from build123d import *

# Parameters (mm, degrees)
SKETCH_1_R          = 1.6
SKETCH_1_W          = 32
SKETCH_1_H          = 32
EXTRUDE_1_DEPTH     = 30
SKETCH_3_W          = 32
SKETCH_3_H          = 32
EXTRUDE_2_DEPTH     = 5
SKETCH_4_R          = 6.35
CUT_EXTRUDE_1_DEPTH = 53.250598083
SKETCH_5_R          = 10
CUT_EXTRUDE_2_DEPTH = 3
CUT_EXTRUDE_3_DEPTH = 3.5
EXTRUDE_3_DEPTH     = 60.5
SKETCH_14_W         = 12.25
SKETCH_14_H         = 14
SKETCH_14_R         = 1.6
EXTRUDE_4_DEPTH     = 4
EXTRUDE_5_DEPTH     = 3
FILLET_1_R          = 1


with BuildPart() as part:
    # ｽｹｯﾁ1 → ﾎﾞｽ - 押し出し1 (new body)
    with BuildSketch(Plane.XY):
        with BuildLine():
            Line((30.25, -30.25), (30.25, 27.25))
            ThreePointArc((30.25, 27.25), (29.371320344, 29.371320344), (27.25, 30.25))
            Line((27.25, 30.25), (-27.25, 30.25))
            ThreePointArc((-27.25, 30.25), (-29.371320344, 29.371320344), (-30.25, 27.25))
            Line((-30.25, 27.25), (-30.25, -30.25))
            Line((-30.25, -30.25), (30.25, -30.25))
        make_face()
        with Locations((-26.25, 26.25)):
            Circle(SKETCH_1_R, mode=Mode.SUBTRACT)
        with Locations((-26.25, -26.25)):
            Circle(SKETCH_1_R, mode=Mode.SUBTRACT)
        with Locations((26.25, -26.25)):
            Circle(SKETCH_1_R, mode=Mode.SUBTRACT)
        with Locations((26.25, 26.25)):
            Circle(SKETCH_1_R, mode=Mode.SUBTRACT)
        Rectangle(SKETCH_1_W, SKETCH_1_H, mode=Mode.SUBTRACT)
    extrude(amount=-EXTRUDE_1_DEPTH)

    # ｽｹｯﾁ3 → ﾎﾞｽ - 押し出し2 (add)
    with BuildSketch(Plane(origin=(0, 0, -30), x_dir=(-1, 0, 0), z_dir=(0, 0, -1))):
        Rectangle(SKETCH_3_W, SKETCH_3_H)
    extrude(amount=-EXTRUDE_2_DEPTH)

    # ｽｹｯﾁ4 → ｶｯﾄ - 押し出し1 (cut, through all)
    with BuildSketch(Plane(origin=(0, 0, -30), x_dir=(-1, 0, 0), z_dir=(0, 0, -1))):
        Circle(SKETCH_4_R)
    extrude(amount=-CUT_EXTRUDE_1_DEPTH, mode=Mode.SUBTRACT)

    # ｽｹｯﾁ5 → ｶｯﾄ - 押し出し2 (cut)
    with BuildSketch(Plane.XY.offset(-25)):
        Circle(SKETCH_5_R)
    extrude(amount=-CUT_EXTRUDE_2_DEPTH, mode=Mode.SUBTRACT)

    # ｽｹｯﾁ10 → ｶｯﾄ - 押し出し3 (cut)
    with BuildSketch(Plane.XY.offset(-4)):
        Polygon((27.895448267, -23.4), (30.25, -23.4), (30.25, -29.1), (27.895448267, -29.1), (24.604551733, -29.1), (22.959103466, -26.25), (24.604551733, -23.4), align=None)
        Polygon((-30.25, -29.1), (-27.895448267, -29.1), (-24.604551733, -29.1), (-22.959103466, -26.25), (-24.604551733, -23.4), (-27.895448267, -23.4), (-30.25, -23.4), align=None)
        Polygon((-27.895448267, 23.4), (-30.25, 23.4), (-30.25, 29.1), (-27.895448267, 29.1), (-24.604551733, 29.1), (-22.959103466, 26.25), (-24.604551733, 23.4), align=None)
        Polygon((30.25, 29.1), (27.895448267, 29.1), (24.604551733, 29.1), (22.959103466, 26.25), (24.604551733, 23.4), (27.895448267, 23.4), (30.25, 23.4), align=None)
    extrude(amount=-CUT_EXTRUDE_3_DEPTH, mode=Mode.SUBTRACT)

    # ｽｹｯﾁ13 → ﾎﾞｽ - 押し出し3 (add)
    with BuildSketch(Plane.ZY.offset(30.25)):
        Polygon((-30, -30.25), (-28.703181865, -36.351049646), (0, -30.25), align=None)
    extrude(amount=-EXTRUDE_3_DEPTH)

    # ｽｹｯﾁ14 → ﾎﾞｽ - 押し出し4 (add)
    with BuildSketch(Plane(origin=(0, -28.942375047, 6.151891727), x_dir=(1, 0, 0), z_dir=(0, -0.9781476007338057, 0.20791169081775968))):
        with Locations((-36.375, -28.633756669)):
            Rectangle(SKETCH_14_W, SKETCH_14_H)
        with Locations(Location((-37.5, -29.633756669, 0), (0, 0, 270))):
            Circle(SKETCH_14_R, mode=Mode.SUBTRACT)
    extrude_4 = extrude(amount=-EXTRUDE_4_DEPTH)

    # ｽｹｯﾁ16 → ﾎﾞｽ - 押し出し5 (add)
    with BuildSketch(Plane(origin=(0, -4.497910928, -21.161007181), x_dir=(1, 0, 0), z_dir=(0, 0.20791169081775962, 0.9781476007338056))):
        Polygon((-42.5, -25.588964922), (-30.25, -13.338964922), (-30.25, -25.588964922), align=None)
    extrude_5 = extrude(amount=-EXTRUDE_5_DEPTH)

    # ﾐﾗｰ1: ﾎﾞｽ - 押し出し4, ﾎﾞｽ - 押し出し5 across plane
    add(extrude_4.mirror(Plane(origin=(0, 0, 0), x_dir=(0, 0, 1), z_dir=(1, 0, 0))))
    add(extrude_5.mirror(Plane(origin=(0, 0, 0), x_dir=(0, 0, 1), z_dir=(1, 0, 0))))

    # ﾌｨﾚｯﾄ1
    fillet_1_edges = [part.edges().sort_by_distance(p)[0] for p in [
        (-30.25, -31.294944944, -24.155016824),
        (-42.5, -34.394754445, -29.119005246),
        (-42.5, -31.483990773, -15.424938836),
        (-36.375, -30.151430644, -18.77520502),
        (-30.25, -24.16027659, -20.048664126),
        (30.25, -31.294944944, -24.155016824),
        (42.5, -31.483990773, -15.424938836),
        (42.5, -34.394754445, -29.119005246),
        (36.375, -30.151430644, -18.77520502),
        (30.25, -24.16027659, -20.048664126),
    ]]
    fillet(fillet_1_edges, radius=FILLET_1_R)


solid = part.part
Design review of the part built by this model. Coordinates are the model's own, in mm. A direction names the side the tool comes from. Coordinates: 2 decimals unless noted, no trailing zeros. Write each loop counter-clockwise with the first axis right and the second up, starting at its lowest first coordinate (ties: lowest second). Pieces come first, ordered by that corner, then holes. Notation, with made-up numbers: (-35.75, 47.25) -> (-3.75, 47.25) arc R18 cw to (-3.75, 62.25) -> close; hole circle Ø1 at (37, -35.75). An arc over 180 degrees is marked (long way). Write each question's results on one line, items separated by ' | '. Start each with the question number.
(1) Take a section at C-C on x = 0. Write out the cut boundary in (y, z), and give its area (3 significant figures).
(2) For line 1 along X through (y, z) = (-5, -23.5); line 2 along Y through (x, z) = (-26, -18); line 3 along Z through (x, y) = (8.5, -7), list the stretches that pass through material, from the lowest coordinate up. Write a range as from..to.
(3) Clearance check with flat-ended pins moving along their axes: P1, Ø1.8, axis at x = -28.5, z = -5.5, coming from the +Y side; P2, Ø8, axis at y = 13.5, z = -12, coming from the +X side; P3, Ø1, axis at y = -24.5, z = -5, coming from the -X side. State where each tip first meets the part, or that it passes through.
(4) The part is to be moulded in two halves that separate along Y. For faces 4 (the face through (-29.35, 29.39, -14.79)), 5 (the face through (0, 21, 0)), 6 (the face through (0, -16, -12)), say which applies: pulls with the +Y half, pulls with the -Y half, needs draft (parallel to the pull), parting line crosses it, or undercut.
(5) Take a section at A-A on x = 26.25. Give the number of separate pieces and of enclosed holes in the cut face, and give its area (3 significant figures).
(6) Tool access review of faces 1 (the face through (23.79, -27.69, -5.73)), 2 (the face through (-16, 0, -12)), 3 (the face through (-23.77, -24.845, -5.726)): name each direction out of +Z, -Z, +X, -X, +Y, -Y from which nothing blocks a thin tool from reaching the whole face with its end or side.
(7) Take a section at B-B on y = 0. Write out the cut boundary in (x, z).
(8) Take a section at D-D on y = -14. Write out the cut boundary in (x, z), and give its area (4 significant figures).
Results found:
1) outline: (-36.35, -28.7) -> (-30.25, -30) -> (-6.35, -30) -> (-6.35, -28) -> (-10, -28) -> (-10, -25) -> (-16, -25) -> (-16, 0) -> (-30.25, 0) -> close; (6.35, -30) -> (30.25, -30) -> (30.25, 0) -> (16, 0) -> (16, -25) -> (10, -25) -> (10, -28) -> (6.35, -28) -> close | area: 1,020 mm2
2) line 1: x = -30.25..-16, 16..30.25 | line 2: y = -34.08..-27.83, -24.67..24.67, 27.83..30.25 | line 3: z = -30..-25
3) P1: stops at y = 30.23 | P2: stops at x = 30.25 | P3: stops at x = -24.26
4) face 4: pulls with the +Y half | face 5: needs draft | face 6: undercut
5) separate pieces: 3 | enclosed holes: 0 | area: 1,700 mm2
6) face 1: +X | face 2: +Z | face 3: -X
7) outline: (-30.25, -30) -> (-6.35, -30) -> (-6.35, -28) -> (-10, -28) -> (-10, -25) -> (-16, -25) -> (-16, 0) -> (-30.25, 0) -> close; (6.35, -30) -> (30.25, -30) -> (30.25, 0) -> (16, 0) -> (16, -25) -> (10, -25) -> (10, -28) -> (6.35, -28) -> close
8) outline: (-30.25, -30) -> (30.25, -30) -> (30.25, 0) -> (16, 0) -> (16, -25) -> (-16, -25) -> (-16, 0) -> (-30.25, 0) -> close | area: 1,015 mm2
